from build123d import *

# Parameters (mm, degrees)
F0_R     = 10
F1_DEPTH = 25
F2_DEPTH = 50
F3_SIZE  = 2
F4_R     = 37.5
F5_DEPTH = 40
F6_SIZE  = 4


with BuildPart() as f1:
    # F0 (on Front) → F1 (new body)
    with BuildSketch(Plane.XZ):
        with BuildLine():
            ThreePointArc((2.083333, -24.913043), (18.399502, -16.92508), (25, 0))
            ThreePointArc((25, 0), (18.399502, 16.92508), (2.083333, 24.913043))
            ThreePointArc((2.083333, 24.913043), (-25, 0), (2.083333, -24.913043))
        make_face()
        Circle(F0_R, mode=Mode.SUBTRACT)
        with BuildLine():
            ThreePointArc((2.083333, 24.913043), (18.399502, 16.92508), (25, 0))
            ThreePointArc((25, 0), (18.399502, -16.92508), (2.083333, -24.913043))
            Line((2.083333, -24.913043), (91.458333, -17.43913))
            ThreePointArc((91.458333, -17.43913), (72.5, 0), (91.458333, 17.43913))
            Line((91.458333, 17.43913), (2.083333, 24.913043))
        make_face()
        with BuildLine():
            ThreePointArc((107.5, 0), (102.879651, 11.847556), (91.458333, 17.43913))
            ThreePointArc((91.458333, 17.43913), (72.5, 0), (91.458333, -17.43913))
            ThreePointArc((91.458333, -17.43913), (102.879651, -11.847556), (107.5, 0))
        make_face()
        with Locations((90, 0)):
            Circle(F0_R, mode=Mode.SUBTRACT)
    extrude(amount=F1_DEPTH)

    # F0 (on Front) → F2 (join)
    with BuildSketch(Plane.XZ):
        with BuildLine():
            ThreePointArc((2.083333, -24.913043), (18.399502, -16.92508), (25, 0))
            ThreePointArc((25, 0), (18.399502, 16.92508), (2.083333, 24.913043))
            ThreePointArc((2.083333, 24.913043), (-25, 0), (2.083333, -24.913043))
        make_face()
        Circle(F0_R, mode=Mode.SUBTRACT)
    extrude(amount=F2_DEPTH)

    # F3
    f3_edges = [f1.edges().sort_by_distance(p)[0] for p in [
        (-2.083333, -50, 24.913043),
        (-10, -50, 0),
        (80, -25, 0),
    ]]
    chamfer(f3_edges, length=F3_SIZE)

    # F4 (on Front) → F5 (join)
    with BuildSketch(Plane.XZ):
        Circle(F4_R)
    extrude(amount=F5_DEPTH)

    # F6
    f6_edges = [f1.edges().sort_by_distance(p)[0] for p in [
        (-37.5, -40, 0),
    ]]
    chamfer(f6_edges, length=F6_SIZE)


solid = f1.part
Design review of the part built by this model. Coordinates are the model's own, in mm. A direction names the side the tool comes from. Give positions to 0.01 mm unless a question says otherwise; leave off trailing zeros. Loops run counter-clockwise (first coordinate to the right, second up) from the corner with the lowest first, then second, coordinate; pieces in that order, holes last. Notation, with made-up numbers: M 84,58 L 93,58 A16 cw 93,87 Z; hole C 28,74.25 d1. An arc over 180 degrees is marked long. One line per question, with ' | ' between items. Start each with the question number.
1. To check wall thickness, follow L1, parallel to Z at x = 0, y = -44.75; L2, parallel to Y at x = 82.5, z = 10. State the ranges of each line that lie inside material, in increasing order.
2. The part is to be moulded in two halves that separate along Z. For faces 1 (the face through (61.128, -12.325, 19.975)), 2 (the face through (81.965, -23.125, -6.161)), 3 (the face through (-13, -40, -22)), say which applies: released by +Z, released by -Z, zero draft, split by the parting line, or undercut.
3. Add section B-B (x = 0). Write out the cut boundary in (y, z).
4. Insertion check: P1, Ø13.5, axis at x = 63.5, z = -8, coming from the -Y side; P2, Ø10, axis at x = 38.5, y = -20, coming from the -Z side; P3, Ø10, axis at y = -28.5, z = -20, coming from the -X side. Each pin has a flat end and moves straight along its axis. Give the tip position at first contact, or say it passes through.
5. Add section C-C (y = -43). Write out the cut boundary in (x, z).
6. Add section D-D (y = -30). Write out the cut boundary in (x, z), plus the area to 3 significant figures.
7. For faces 4 (the face through (60.267, -12.325, -20.047)), 5 (the face through (0, -40, 0)), list the 3-axis set-ups (+Z, -Z, +X, -X, +Y, -Y) from which the entire face can be reached by the end or side of a thin tool; tool diameter is ignored.
8. Add section A-A (y = -15). Write out the cut boundary in (x, z).
Worked out:
1) L1: z = -25 to -10, 10 to 25 | L2: y = -25 to 0
2) face 1: released by +Z | face 2: undercut | face 3: zero draft
3) outline: M -50,-23 L -48,-25 L -40,-25 L -40,-33.5 L -36,-37.5 L 0,-37.5 L 0,37.5 L -36,37.5 L -40,33.5 L -40,25 L -48,25 L -50,23 L -50,12 L -48,10 L -40,10 L -40,-10 L -48,-10 L -50,-12 Z
4) P1: stops at y = -25 | P2: stops at z = -22.29 | P3: stops at x = -34.37
5) outline: M 2.08,-24.91 A25 ccw 25,0 A25 ccw 2.08,24.91 A25 ccw long Z; hole C 0,0 d20
6) outline: C 0,0 d75 | area: 4,420 mm²
7) face 4: -Z, +X, +Y, -Y | face 5: -Y
8) outline: M 29.94,-22.58 L 91.46,-17.44 A17.5 ccw 91.46,17.44 L 29.94,22.58 A37.5 ccw long Z; hole C 90,0 d20
